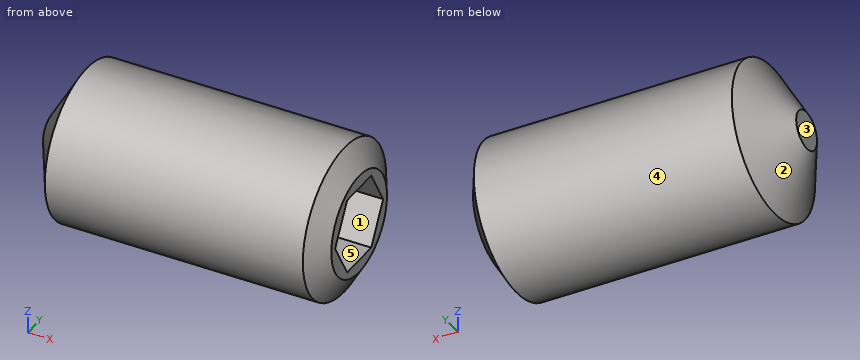
Autodesk Inventor part; units mm, degrees
ref_plane "Work Plane1" through (8, 0, 0) normal (0, 0, 1) x (1, 0, 0)
ref_plane "YZ Plane" through (0, 0, 0) normal (1, 0, 0) x (0, 1, 0)
ref_plane "XZ Plane" through (0, 0, 0) normal (0, 1, 0) x (-1, 0, 0)
sketch "Эскиз1" plane through (0, 0, 0) normal (0, 0, 1) x (1, 0, 0)
  line L0 (0, 0) -> (9.6667, 0)
  line L1 (16, 2.3094) -> (16, 4)
  line L2 (16, 4) -> (0, 4)
  line L3 (16, 2.3094) -> (11, 2.3094)
  line L4 (11, 2.3094) -> (9.6667, 0)
  line L5 (0, -0.8) -> (0, 4.8)
  line L6 (0, 4) -> (0, 0)
  dimension "d0" = 5
  dimension "d1" = 60
  dimension "d2" = 8
  dimension "d3" = 4.6188
  dimension "d5" = 16
revolve "Базовый элемент" add sketch "Эскиз1" angle 360 about axis through (0, 0, 0) along (1, 0, 0)
sketch "Эскиз2" plane through (16, 0, 0) normal (1, 0, 0) x (0, 1, 0)
  circle A0 centre (0, 0) radius 2.3094
  line L0 (-1.1547, 2) -> (1.1547, 2)
  line L1 (1.1547, 2) -> (2.3094, 0)
  line L2 (2.3094, 0) -> (1.1547, -2)
  line L3 (1.1547, -2) -> (-1.1547, -2)
  line L4 (-1.1547, -2) -> (-2.3094, 0)
  line L5 (-2.3094, 0) -> (-1.1547, 2)
  point P0 (0, 0)
  point P1 (0, 0)
extrude "Паз" add sketch "Эскиз2" against normal up to next contours L1 A0 | A0 L2 | L0 A0 | A0 L3 | L5 A0 | A0 L4
thread "Резьба"
chamfer "Фаска1" distance 1.7321 angle 60 1 edges at (0, -4, 0) measured on face at (10.6667, 3.987, -0.3219)
chamfer "Фаска2" distance 0.7668 angle 60 1 edges at (16, -4, 0) measured on face at (11.244, 3.9482, -0.6416)
ref_plane "Work Plane1" through (8, 0, 0) normal (0, 0, 1) x (1, 0, 0)
equation "\"d0\" = INTI"
equation "\"d2\" = NND"
equation "\"d3\" = 1.1547 * SW"
equation "\"d5\" = NLG"
equation "\"d12\" = NLG"
equation "\"d9\" = FAWI"
equation "\"d10\" = -0.5 * GD1 + 0.5 * NND"
equation "\"d11\" = FAWI"
equation "\"d35\" = -0.5 * GD1 + 0.5 * NND"
equation "\"NND\" = 8"
equation "\"NLG\" = 16"
equation "\"INTI\" = 5"
equation "\"FAWI\" = 60deg"
equation "\"SW\" = 4"
equation "\"GD1\" = THREADDIA - 1.2269 * PTC"
equation "\"FAWI1\" = 45deg"
equation "\"SPD\" = 2"
equation "\"GUL\" = 0.61345 * PTC"
equation "\"TOA\" = 30deg"
equation "\"THREADDIA\" = 8"
equation "\"PTC\" = 1.25"
equation "\"GAL\" = 0.61345 * PTC"
equation "\"E0\" = 1.155 * SW"
properties part number "AS 1421 - M8x16 конический" material "Сталь, мягкая"
Here's how the part is built. I have some questions about the finished solid (model axes, mm). Face numbers are marked on the shaded views. A direction names the side the tool comes from. Coordinates: 2 decimals unless noted, no trailing zeros. Order: outer loops, then holes, each group sorted by start corner. A loop starts at its lowest first (then second) coordinate and runs counter-clockwise, first axis right, second up.
1) Which directions (+Z, -Z, +X, -X, +Y, -Y) give clear straight access to the entire face, cutting with the end or side of a thin tool? Please do the marked faces 4 and 5.
2) I need wall thicknesses on line 1 (Y direction, x = 14.25, z = 1); line 2 (Z direction, x = 12, y = -0.5); line 3 (Z direction, x = 14.5, y = -1.5). Which ranges of each line are inside material? Lowest first, please.
3) We'd pull the mould along Y, two halves only. Please class the marked faces 1, 2 and 3: +Y half, -Y half, draft (parallel to the pull), parting line (faces both ways), or undercut.
4) Will this pin go through, and if not, where does the flat tip stop? pin 1 (1 mm diameter, centred on x = 4, y = -2, fed in from +Z).
5) Imagine slicing it at A-A on x = 12. List the corners of the cut face in (y, z) for me.
6) Imagine slicing it at B-B on x = 9.5. List the corners of the cut face in (y, z) for me, and give its area (3 significant figures).
Response values:
1. face 4: +X, -X
1. face 5: +X
2. line 1: y = -3.87 to -1.73, 1.73 to 3.87
2. line 2: z = -3.97 to -2, 2 to 3.97
2. line 3: z = -3.71 to -1.4, 1.4 to 3.71
3. face 1: undercut
3. face 2: parting line
3. face 3: draft
4. pin 1: stops at z = 3.71
5. outline: circle Ø8 at (0, 0); hole (-2.31, 0) - (-1.15, -2) - (1.15, -2) - (2.31, 0) - (1.15, 2) - (-1.15, 2) - close
6. outline: circle Ø8 at (0, 0)
6. area: 50.3 mm2
